Can you work these out from the model? Positions are in its coordinate system, mm. A direction names the side the tool comes from. Give positions to 0.01 mm unless a question says otherwise; leave off trailing zeros. Write each loop counter-clockwise with the first axis right and the second up, starting at its lowest first coordinate (ties: lowest second). Pieces come first, ordered by that corner, then holes.
from build123d import *

# Parameters (mm, degrees)
F0_W     = 83
F0_H     = 71
F1_DEPTH = 25
F2_W     = 67
F2_H     = 61
F3_DEPTH = 20
F4_W     = 5.2
F4_H     = 52
F5_DEPTH = 25.001


with BuildPart() as f1:
    # F0 (on Top) → F1 (new body)
    with BuildSketch(Plane.XY):
        Rectangle(F0_W, F0_H)
    extrude(amount=F1_DEPTH)

    # F2 (on face) → F3 (cut)
    with BuildSketch(Plane.XY.offset(25)):
        Rectangle(F2_W, F2_H)
    extrude(amount=-F3_DEPTH, mode=Mode.SUBTRACT)

    # F4 (on Top) → F5 (cut, through all)
    with BuildSketch(Plane.XY):
        with Locations((-26.9, 0.5)):
            Rectangle(F4_W, F4_H)
    extrude(amount=F5_DEPTH, mode=Mode.SUBTRACT)


solid = f1.part
(1) Will this pin go through, and if not, where does the flat tip stop? P1, Ø12, axis at x = 24.5, y = 2.5, coming from the -Z side.
Returned:
P1: stops at z = 0
(2) Imagine slicing it at B-B, the plane x = -25.5. Write out the boundary of the cut face in (y, z).
Returned:
outline: (-35.5, 0) - (-25.5, 0) - (-25.5, 5) - (-30.5, 5) - (-30.5, 25) - (-35.5, 25) - close; (26.5, 0) - (35.5, 0) - (35.5, 25) - (30.5, 25) - (30.5, 5) - (26.5, 5) - close
(3) If we mould it in two halves opening along Y, with no side actions, what happens to faces 4 (the face through (-1, -35.5, 12)), 5 (the face through (-41.5, 0, 12)), 6 (the face through (-27, -25.5, 2))? For each: +Y half, -Y half, draft (parallel to the pull), parting line (faces both ways), or undercut.
Returned:
face 4: -Y half
face 5: draft
face 6: undercut
(4) If I drill on L1, parallel to Y at x = -18.5, z = 9; L2, parallel to X at y = 26, z = 17.75; L3, parallel to X at y = -5, z = 4.75, over which ranges is the centre line in solid material (lowest first)?
Returned:
L1: y = -35.5 to -30.5, 30.5 to 35.5
L2: x = -41.5 to -33.5, 33.5 to 41.5
L3: x = -41.5 to -29.5, -24.3 to 41.5
(5) Imagine slicing it at D-D, the plane y = -29. Write out the boundary of the cut face in (x, z), plus the area to 3 significant figures.
Returned:
outline: (-41.5, 0) - (41.5, 0) - (41.5, 25) - (33.5, 25) - (33.5, 5) - (-33.5, 5) - (-33.5, 25) - (-41.5, 25) - close
area: 735 mm2
(6) For faces 1 (the face through (33.5, 0, 15)), 2 (the face through (-24.3, 0, 2)), 3 (the face through (-1, 35.5, 12)), which set-ups out of +Z, -Z, +X, -X, +Y, -Y let a thin tool reach every point of the face, with its end or its side?
Returned:
face 1: +Z
face 2: +Z, -Z
face 3: +Z, -Z, +X, -X, +Y
(7) Imagine slicing it at A-A, the plane y = 2. Write out the boundary of the cut face in (x, z).
Returned:
outline: (-41.5, 0) - (-29.5, 0) - (-29.5, 5) - (-33.5, 5) - (-33.5, 25) - (-41.5, 25) - close; (-24.3, 0) - (41.5, 0) - (41.5, 25) - (33.5, 25) - (33.5, 5) - (-24.3, 5) - close
(8) Imagine slicing it at C-C, the plane z = 16.25. Write out the boundary of the cut face in (x, y).
Returned:
outline: (-41.5, -35.5) - (41.5, -35.5) - (41.5, 35.5) - (-41.5, 35.5) - close; hole (-33.5, -30.5) - (33.5, -30.5) - (33.5, 30.5) - (-33.5, 30.5) - close
